```python
from build123d import *

# Parameters (mm, degrees)
PAD_DEPTH       = 4
SKETCH001_R     = 2
POCKET_DEPTH    = 4.001
SKETCH002_R     = 2
POCKET001_DEPTH = 4.001
SKETCH003_R     = 1
POCKET002_DEPTH = 4.001
SKETCH004_R     = 1
POCKET003_DEPTH = 4.001
SKETCH005_W     = 22
SKETCH005_H     = 5
PAD001_DEPTH    = 15
POCKET004_DEPTH = 50.001
FILLET_R        = 2
FILLET001_R     = 2
FILLET002_R     = 2
FILLET003_R     = 2
FILLET004_R     = 2
SKETCH007_W     = 17
SKETCH007_H     = 4
POCKET005_DEPTH = 2
PAD002_DEPTH    = 3


with BuildPart() as part:
    # Sketch → Pad (new body)
    with BuildSketch(Plane.XY):
        Polygon((-20, 20), (20, 20), (20, 0), (0, 0), (0, -30), (-20, -30), align=None)
    extrude(amount=PAD_DEPTH)

    # Sketch001 (on Face8 of Pad) → Pocket (cut, through all)
    with BuildSketch(Plane.XY.offset(4)):
        with Locations((-10, 15)):
            Circle(SKETCH001_R)
    extrude(amount=-POCKET_DEPTH, mode=Mode.SUBTRACT)

    # Sketch002 (on Face5 of Pocket) → Pocket001 (cut, through all)
    with BuildSketch(Plane.XY.offset(4)):
        with Locations((-10, 0)):
            Circle(SKETCH002_R)
    extrude(amount=-POCKET001_DEPTH, mode=Mode.SUBTRACT)

    # Sketch003 (on Face5 of Pocket001) → Pocket002 (cut, through all)
    with BuildSketch(Plane.XY.offset(4)):
        with Locations((2.5, 4)):
            Circle(SKETCH003_R)
    extrude(amount=-POCKET002_DEPTH, mode=Mode.SUBTRACT)

    # Sketch004 (on Face5 of Pocket002) → Pocket003 (cut, through all)
    with BuildSketch(Plane.XY.offset(4)):
        with Locations((17.5, 4)):
            Circle(SKETCH004_R)
    extrude(amount=-POCKET003_DEPTH, mode=Mode.SUBTRACT)

    # Sketch005 (on Face5 of Pocket003) → Pad001 (join)
    with BuildSketch(Plane.XY.offset(4)):
        with Locations((5, 17.5)):
            Rectangle(SKETCH005_W, SKETCH005_H)
    extrude(amount=PAD001_DEPTH)

    # Sketch006 (on Face6 of Pad001) → Pocket004 (cut, through all)
    with BuildSketch(Plane(origin=(0, 20, 0), x_dir=(-1, 0, 0), z_dir=(0, 1, 0))):
        with BuildLine():
            ThreePointArc((-5, 15.5), (-9.5, 11), (-5, 6.5))
            Line((-5, 6.5), (0, 6.5))
            ThreePointArc((0, 6.5), (4.5, 11), (0, 15.5))
            Line((-5, 15.5), (0, 15.5))
        make_face()
    extrude(amount=-POCKET004_DEPTH, mode=Mode.SUBTRACT)

    # Fillet
    fillet_edges = [part.edges().sort_by_distance(p)[0] for p in [
        (20, 0, 2),
    ]]
    fillet(fillet_edges, radius=FILLET_R)

    # Fillet001
    fillet001_edges = [part.edges().sort_by_distance(p)[0] for p in [
        (20, 20, 2),
    ]]
    fillet(fillet001_edges, radius=FILLET001_R)

    # Fillet002
    fillet002_edges = [part.edges().sort_by_distance(p)[0] for p in [
        (-20, 20, 2),
    ]]
    fillet(fillet002_edges, radius=FILLET002_R)

    # Fillet003
    fillet003_edges = [part.edges().sort_by_distance(p)[0] for p in [
        (-6, 17.5, 19),
    ]]
    fillet(fillet003_edges, radius=FILLET003_R)

    # Fillet004
    fillet004_edges = [part.edges().sort_by_distance(p)[0] for p in [
        (16, 17.5, 19),
    ]]
    fillet(fillet004_edges, radius=FILLET004_R)

    # Sketch007 (on Face13 of Fillet004) → Pocket005 (cut)
    with BuildSketch(Plane.XY.offset(4)):
        with Locations((2.5, 13)):
            Rectangle(SKETCH007_W, SKETCH007_H)
    extrude(amount=-POCKET005_DEPTH, mode=Mode.SUBTRACT)

    # Sketch008 (on Face5 of Pocket005) → Pad002 (join)
    with BuildSketch(Plane.YZ.offset(16)):
        Polygon((15, 4), (8, 4), (8, 9), (13, 16), (15, 16), align=None)
    extrude(amount=-PAD002_DEPTH)


solid = part.part
```
CAD build for the part. Positions are in the model's coordinates, mm. A direction names the side the tool comes from. Give positions to 0.01 mm unless a question says otherwise; leave off trailing zeros. Write each loop counter-clockwise with the first axis right and the second up, starting at its lowest first coordinate (ties: lowest second). Pieces come first, ordered by that corner, then holes. Notation, with made-up numbers: M 41.25,-24 L 97.25,-24 A29 cw 97.25,4 Z; hole C -14,63 d4. An arc over 180 degrees is marked long. Return JSON: item names as keys, results as strings. Group by question number.
(1) Band-saw the part on B-B (x = 7). Give the cut face in (y, z).
(2) 3-axis set-ups, long thin cutter, end or side, ignore diameter. For faces 1 (the face through (9, 0, 2)), 2 (the face through (9.5, 17.5, 11.1)), 3 (the face through (15, 14, 16)), 4 (the face through (16, 15, 9)), 5 (the face through (11, 13, 3)): which of +Z, -Z, +X, -X, +Y, -Y reach the whole face in a straight line?
(3) Drill centre lines: L1, parallel to Y at x = -10, z = 2.5; L2, parallel to Y at x = 17.5, z = 2.95; L3, parallel to Z at x = -11.5, y = 8. Where is each one in solid material? Low to high. Write a range as [from, to].
(4) Band-saw the part on A-A (y = 4). Give the cut face in (x, z), and give its area (3 significant figures).
(5) Band-saw the part on D-D (x = -9). Give the cut face in (y, z).
(6) Band-saw the part on C-C (z = 11). Give the cut face in (x, y), and give its area (3 significant figures).
(7) Mould opens along X. For faces 6 (the face through (13, 12, 9)), 7 (the face through (3, 18, 6.5)), 8 (the face through (19.43, 0.6, 2.03)), 9 (the face through (3, 18, 15.5)) say: pulls with the +X half, pulls with the -X half, needs draft (parallel to the pull), parting line crosses it, or undercut.
(8) Flat gauge pins, fed straight in: pin 1 Ø1.5 at (y, z) = (16.5, 11) entering from -X; pin 2 Ø4.5 at (y, z) = (-11.5, 1) entering from +X; pin 3 Ø4 at (y, z) = (9.5, 10) entering from -X. Where does each tip first touch, or does it go through?
Entries:
{
 "1": {"outline": "M 0,0 L 20,0 L 20,6.97 L 15,6.97 L 15,2 L 11,2 L 11,4 L 0,4 Z; M 15,15.03 L 20,15.03 L 20,19 L 15,19 Z"},
 "2": {"face 1": "+Z, -Z, +X, -Y", "face 2": "+Y, -Y", "face 3": "+Z, +X, -X, -Y", "face 4": "+Z, +X, +Y, -Y", "face 5": "+Z"},
 "3": {"L1": "y = [-30, -2], [2, 13], [17, 20]", "L2": "y = [0, 3], [5, 20]", "L3": "z = [0, 4]"},
 "4": {"outline": "M -20,0 L 1.5,0 L 1.5,4 L -20,4 Z; M 3.5,0 L 16.5,0 L 16.5,4 L 3.5,4 Z; M 18.5,0 L 20,0 L 20,4 L 18.5,4 Z", "area": "144 mm^2"},
 "5": {"outline": "M -30,0 L -1.73,0 L -1.73,4 L -30,4 Z; M 1.73,0 L 13.27,0 L 13.27,4 L 1.73,4 Z; M 16.73,0 L 20,0 L 20,4 L 16.73,4 Z"},
 "6": {"outline": "M -6,15 L -4.5,15 L -4.5,20 L -6,20 Z; M 9.5,15 L 13,15 L 13,9.43 L 16,9.43 L 16,20 L 9.5,20 Z", "area": "56.7 mm^2"},
 "7": {"face 6": "pulls with the -X half", "face 7": "undercut", "face 8": "pulls with the +X half", "face 9": "undercut"},
 "8": {"pin 1": "stops at x = -6", "pin 2": "stops at x = 0", "pin 3": "stops at x = 13"}
}
